```python
from build123d import *

# Parameters (mm, degrees)
SKETCH1_W               = 279.4
SKETCH1_H               = 279.4
BOSS_EXTRUDE1_DEPTH     = 12.7
SKETCH2_W               = 25.4
SKETCH2_H               = 12.7
BOSS_EXTRUDE2_DEPTH     = 12.7
LPATTERN1_COUNT         = 6
LPATTERN1_PITCH         = 50.8
MIRROR1_COPY_1_SKETCH_W = 25.4
MIRROR1_COPY_1_SKETCH_H = 12.7
MIRROR1_COPY_1_DEPTH    = 12.7
MIRROR1_COPY_2_SKETCH_W = 25.4
MIRROR1_COPY_2_SKETCH_H = 12.7
MIRROR1_COPY_2_DEPTH    = 12.7
MIRROR1_COPY_3_SKETCH_W = 25.4
MIRROR1_COPY_3_SKETCH_H = 12.7
MIRROR1_COPY_3_DEPTH    = 12.7
MIRROR1_COPY_4_SKETCH_W = 25.4
MIRROR1_COPY_4_SKETCH_H = 12.7
MIRROR1_COPY_4_DEPTH    = 12.7
MIRROR1_COPY_5_SKETCH_W = 25.4
MIRROR1_COPY_5_SKETCH_H = 12.7
MIRROR1_COPY_5_DEPTH    = 12.7
SKETCH3_W               = 25.4
SKETCH3_H               = 12.7
BOSS_EXTRUDE3_DEPTH     = 12.7
LPATTERN2_COUNT         = 6
LPATTERN2_PITCH         = 50.8
SKETCH5_W               = 25.4
SKETCH5_H               = 12.7
BOSS_EXTRUDE4_DEPTH     = 12.7
SKETCH6_R               = 2.1
CUT_EXTRUDE1_DEPTH      = 13.7
SKETCH7_R               = 4.318
CUT_EXTRUDE2_DEPTH      = 6.35
SKETCH8_R               = 2.2225
CUT_EXTRUDE3_DEPTH      = 13.7
SKETCH9_R               = 6.35
CUT_EXTRUDE4_DEPTH      = 6.35
CUT_EXTRUDE5_DEPTH      = 13.7
CUT_EXTRUDE6_DEPTH      = 6.35


with BuildPart() as part:
    # Sketch1 → Boss-Extrude1 (new body)
    with BuildSketch(Plane(origin=(0, 0, 0), x_dir=(1, 0, 0), z_dir=(0, 1, 0))):
        Rectangle(SKETCH1_W, SKETCH1_H)
    extrude(amount=BOSS_EXTRUDE1_DEPTH)

    # Sketch2 → Boss-Extrude2 (add)
    with BuildSketch(Plane(origin=(139.7, 0, 0), x_dir=(0, 0, -1), z_dir=(1, 0, 0))):
        with Locations((-127, 6.35)):
            Rectangle(SKETCH2_W, SKETCH2_H)
    boss_extrude2 = extrude(amount=BOSS_EXTRUDE2_DEPTH)

    # LPattern1: Boss-Extrude2 ×6
    with Locations(*[(0, 0, -i * LPATTERN1_PITCH) for i in range(1, LPATTERN1_COUNT)]):
        add(boss_extrude2)

    # Mirror1: Boss-Extrude2 across plane
    add(boss_extrude2.mirror(Plane(origin=(0, 0, 0), x_dir=(0, 0, 1), z_dir=(1, 0, 0))))

    # Mirror1 copy 1 sketch → Mirror1 copy 1 (add)
    with BuildSketch(Plane(origin=(-139.7, 0, -50.8), x_dir=(0, 0, -1), z_dir=(-1, 0, 0))):
        with Locations((-127, -6.35)):
            Rectangle(MIRROR1_COPY_1_SKETCH_W, MIRROR1_COPY_1_SKETCH_H)
    extrude(amount=MIRROR1_COPY_1_DEPTH)

    # Mirror1 copy 2 sketch → Mirror1 copy 2 (add)
    with BuildSketch(Plane(origin=(-139.7, 0, -101.6), x_dir=(0, 0, -1), z_dir=(-1, 0, 0))):
        with Locations((-127, -6.35)):
            Rectangle(MIRROR1_COPY_2_SKETCH_W, MIRROR1_COPY_2_SKETCH_H)
    extrude(amount=MIRROR1_COPY_2_DEPTH)

    # Mirror1 copy 3 sketch → Mirror1 copy 3 (add)
    with BuildSketch(Plane(origin=(-139.7, 0, -152.4), x_dir=(0, 0, -1), z_dir=(-1, 0, 0))):
        with Locations((-127, -6.35)):
            Rectangle(MIRROR1_COPY_3_SKETCH_W, MIRROR1_COPY_3_SKETCH_H)
    extrude(amount=MIRROR1_COPY_3_DEPTH)

    # Mirror1 copy 4 sketch → Mirror1 copy 4 (add)
    with BuildSketch(Plane(origin=(-139.7, 0, -203.2), x_dir=(0, 0, -1), z_dir=(-1, 0, 0))):
        with Locations((-127, -6.35)):
            Rectangle(MIRROR1_COPY_4_SKETCH_W, MIRROR1_COPY_4_SKETCH_H)
    extrude(amount=MIRROR1_COPY_4_DEPTH)

    # Mirror1 copy 5 sketch → Mirror1 copy 5 (add)
    with BuildSketch(Plane(origin=(-139.7, 0, -254), x_dir=(0, 0, -1), z_dir=(-1, 0, 0))):
        with Locations((-127, -6.35)):
            Rectangle(MIRROR1_COPY_5_SKETCH_W, MIRROR1_COPY_5_SKETCH_H)
    extrude(amount=MIRROR1_COPY_5_DEPTH)

    # Sketch3 → Boss-Extrude3 (add)
    with BuildSketch(Plane(origin=(0, 0, -139.7), x_dir=(-1, 0, 0), z_dir=(0, 0, -1))):
        with Locations((-130.175, 6.35)):
            Rectangle(SKETCH3_W, SKETCH3_H)
    boss_extrude3 = extrude(amount=BOSS_EXTRUDE3_DEPTH)

    # LPattern2: Boss-Extrude3 ×6
    with Locations(*[(-i * LPATTERN2_PITCH, 0, 0) for i in range(1, LPATTERN2_COUNT)]):
        add(boss_extrude3)

    # Sketch5 → Boss-Extrude4 (add)
    with BuildSketch(Plane(origin=(0, 0, -139.7), x_dir=(-1, 0, 0), z_dir=(0, 0, -1))):
        with Locations((-139.7, 6.35)):
            Rectangle(SKETCH5_W, SKETCH5_H)
    boss_extrude4 = extrude(amount=BOSS_EXTRUDE4_DEPTH)

    # Mirror2: Boss-Extrude4 across plane
    add(boss_extrude4.mirror(Plane(origin=(0, 0, 0), x_dir=(0, 0, 1), z_dir=(1, 0, 0))))

    # Sketch6 → Cut-Extrude1 (cut, through all)
    with BuildSketch(Plane.XZ):
        with Locations((44.45, -58.145648771)):
            Circle(SKETCH6_R)
        with Locations((31.75, -46.715648771)):
            Circle(SKETCH6_R)
        with Locations((31.75, 95.524351229)):
            Circle(SKETCH6_R)
        with Locations((44.45, 84.094351229)):
            Circle(SKETCH6_R)
    extrude(amount=-CUT_EXTRUDE1_DEPTH, mode=Mode.SUBTRACT)

    # Sketch7 → Cut-Extrude2 (cut)
    with BuildSketch(Plane.XZ):
        with Locations((31.75, 95.524351229)):
            Circle(SKETCH7_R)
        with Locations((44.45, 84.094351229)):
            Circle(SKETCH7_R)
        with Locations((31.75, -46.715648771)):
            Circle(SKETCH7_R)
        with Locations((44.45, -58.145648771)):
            Circle(SKETCH7_R)
    extrude(amount=-CUT_EXTRUDE2_DEPTH, mode=Mode.SUBTRACT)

    # Sketch8 → Cut-Extrude3 (cut, through all)
    with BuildSketch(Plane(origin=(0, 12.7, 0), x_dir=(1, 0, 0), z_dir=(0, 1, 0))):
        with Locations((-49.920301731, -19.083881859)):
            Circle(SKETCH8_R)
        with Locations((-44.920301731, -9.083881859)):
            Circle(SKETCH8_R)
        with Locations((-94.920301731, -19.083881859)):
            Circle(SKETCH8_R)
        with Locations((-99.920301731, -9.083881859)):
            Circle(SKETCH8_R)
    extrude(amount=-CUT_EXTRUDE3_DEPTH, mode=Mode.SUBTRACT)

    # Sketch9 → Cut-Extrude4 (cut)
    with BuildSketch(Plane.XZ):
        with Locations((-94.920301731, 19.083881859)):
            Circle(SKETCH9_R)
        with Locations((-49.920301731, 19.083881859)):
            Circle(SKETCH9_R)
    extrude(amount=-CUT_EXTRUDE4_DEPTH, mode=Mode.SUBTRACT)

    # Sketch10 → Cut-Extrude5 (cut, through all)
    with BuildSketch(Plane.XZ):
        with BuildLine():
            Line((-112.628282809, 11.348870188), (-32.184656299, 11.348870188))
            ThreePointArc((-32.184656299, 11.348870188), (-29.919667971, 9.083881859), (-32.184656299, 6.81889353))
            Line((-32.184656299, 6.81889353), (-112.628282809, 6.81889353))
            ThreePointArc((-112.628282809, 6.81889353), (-114.893271138, 9.083881859), (-112.628282809, 11.348870188))
        make_face()
        with BuildLine():
            Line((-107.547672787, 28.200110176), (-37.142684893, 28.200110176))
            ThreePointArc((-37.142684893, 28.200110176), (-28.026456576, 19.083881859), (-37.142684893, 9.967653542))
            Line((-37.142684893, 9.967653542), (-107.547672787, 9.967653542))
            ThreePointArc((-107.547672787, 9.967653542), (-116.663901104, 19.083881859), (-107.547672787, 28.200110176))
        make_face()
    extrude(amount=-CUT_EXTRUDE5_DEPTH, mode=Mode.SUBTRACT)

    # Sketch12 → Cut-Extrude6 (cut)
    with BuildSketch(Plane.XZ):
        with BuildLine():
            Line((-107.547672787, 32.464365023), (-37.791668277, 32.464365023))
            ThreePointArc((-37.791668277, 32.464365023), (-24.411185114, 19.083881859), (-37.791668277, 5.703398696))
            Line((-37.791668277, 5.703398696), (-107.547672787, 5.703398696))
            ThreePointArc((-107.547672787, 5.703398696), (-120.92815595, 19.083881859), (-107.547672787, 32.464365023))
        make_face()
    extrude(amount=-CUT_EXTRUDE6_DEPTH, mode=Mode.SUBTRACT)


solid = part.part
```
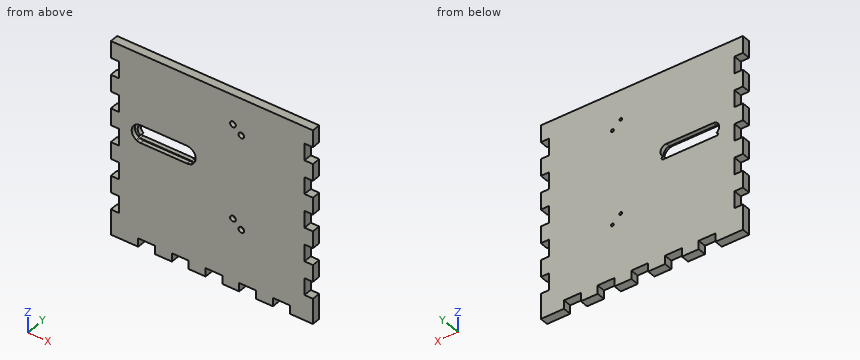
Input: part model. Units: mm. Frame: model coordinates. Give positions to 0.01 mm unless a question says otherwise; leave off trailing zeros. Order: outer loops, then holes, each group sorted by start corner. A loop starts at its lowest first (then second) coordinate and runs counter-clockwise, first axis right, second up. Notation, with made-up numbers: M -1,36 L 7,36 A32 cw 7,68 Z; hole C 39.25,-21 d11. An arc over 180 degrees is marked long. Return JSON: item names as keys, results as strings.
1) Line query: L1, parallel to Z at x = 31.75, y = 4; L2, parallel to Z at x = 31.75, y = 8; L3, parallel to Z at x = -92, y = 1.75. Output: solid intervals per line, ascending. Write a range as [from, to].
Taken from the geometry:
{"L1": "z = [-152.4, -51.03], [-42.4, 91.21], [99.84, 139.7]", "L2": "z = [-152.4, -48.82], [-44.62, 93.42], [97.62, 139.7]", "L3": "z = [-139.7, 5.7], [32.46, 139.7]"}
2) Section query A-A on z = 103.5. Output: boundary loops of the cut face in (x, y), and give its area (3 significant figures).
Taken from the geometry:
{"outline": "M -139.7,0 L 139.7,0 L 139.7,12.7 L -139.7,12.7 Z", "area": "3,550 mm2"}
3) Contact query for flat-ended pins moving along their axis: pin 1 (5 mm diameter, centred on x = 44.45, z = -58.15, fed in from -Y); pin 2 (6.5 mm diameter, centred on x = 2.5, y = 8, fed in from -Z); pin 3 (6.5 mm diameter, centred on y = 5.5, z = -103, fed in from -X); pin 4 (4 mm diameter, centred on x = -106, z = 64, fed in from -Y). Output: stop coordinate, or through.
Taken from the geometry:
{"pin 1": "stops at y = 6.35", "pin 2": "stops at z = -139.7", "pin 3": "stops at x = -139.7", "pin 4": "stops at y = 0"}
4) Section query C-C on x = 109. Output: boundary loops of the cut face in (y, z).
Taken from the geometry:
{"outline": "M 0,-139.7 L 12.7,-139.7 L 12.7,139.7 L 0,139.7 Z"}
5) Section query B-B on y = 4.25. Count the separate pieces of the cut face and the enclosed holes in it, and give its area (3 significant figures).
Taken from the geometry:
{"separate pieces": "1", "enclosed holes": "5", "area": "81,500 mm2"}
